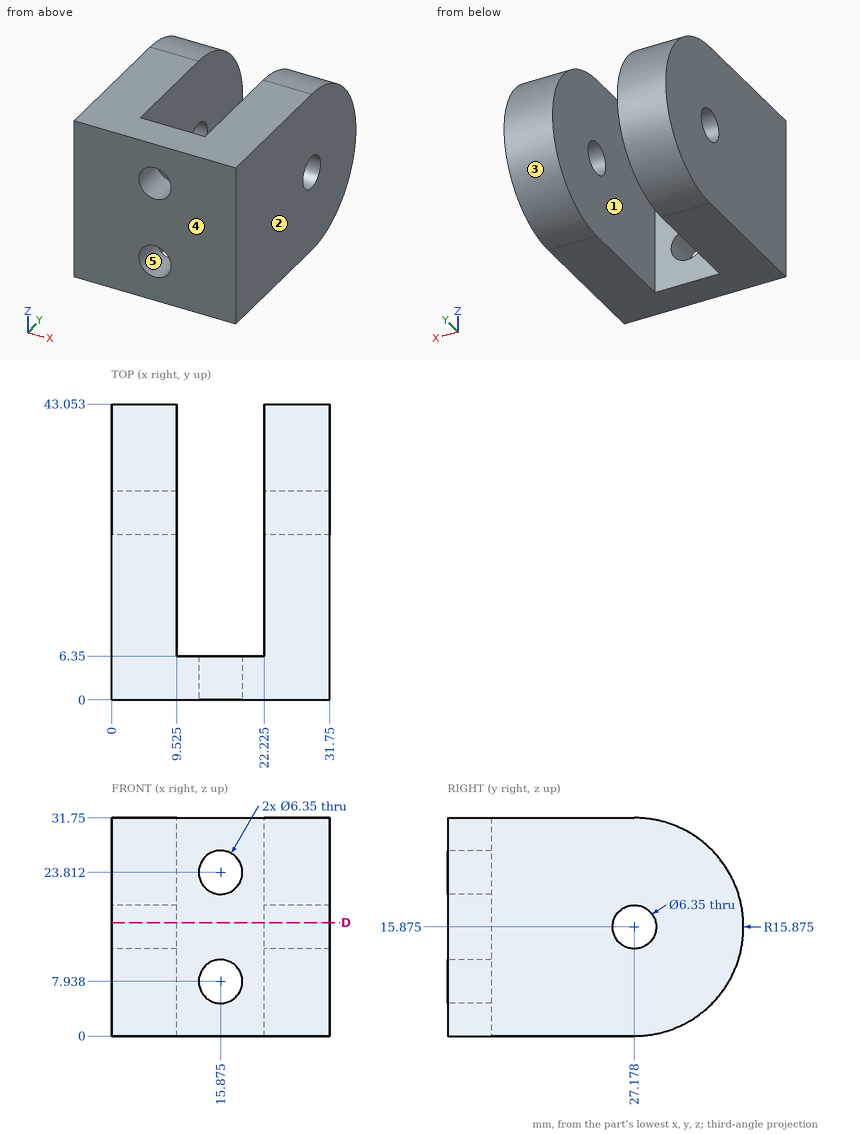
Geometry check sheet. Reference: drawing and pictorial views, mm from the part's lowest x, y, z. A direction names the side the tool comes from. Round coordinates to 2 decimals unless told otherwise and drop trailing zeros. Answer as a JSON object with one key per item and string values. Group by question number.
Item 1: Release check for a two-part mould opening along Z. For the marked faces 3, 4 and 5 record: pulls with the +Z half, pulls with the -Z half, needs draft (parallel to the pull), parting line crosses it, or undercut.
Item 2: Cross-section at D-D, the plane z = 16.5. Count the separate pieces of the cut face and the enclosed holes in it, plus the area to 3 significant figures.
Item 3: Thickness scan on line 1 along Y through (x, z) = (4, 13) (1 decimal); line 2 along Y through (x, z) = (12, 21); line 3 along Y through (x, z) = (24.5, 16.5) (1 decimal). Record the ranges inside material, lowest first.
Item 4: Set-up check for the marked faces 1 and 2: record each of +Z, -Z, +X, -X, +Y, -Y from which the full face is reachable in a straight line by a thin tool's end or side.
Item 5: Depth check by flat-ended pin: pin 1 Ø8 at (x, z) = (11.5, 25) entering from -Y; pin 2 Ø8.5 at (x, z) = (15.88, 7.94) entering from +Y. Enter the tip coordinate at first touch or a pass-through.
Determined:
{
 "1": {"face 3": "parting line crosses it", "face 4": "needs draft", "face 5": "undercut"},
 "2": {"separate pieces": "3", "enclosed holes": "0", "area": "782 mm²"},
 "3": {"line 1": "y = 0 to 25.8, 28.5 to 42.8", "line 2": "y = 0 to 6.35", "line 3": "y = 0 to 24.1, 30.3 to 43"},
 "4": {"face 1": "+Z, -Z, +Y", "face 2": "+Z, -Z, +X, +Y, -Y"},
 "5": {"pin 1": "stops at y = 0", "pin 2": "stops at y = 6.35"}
}
